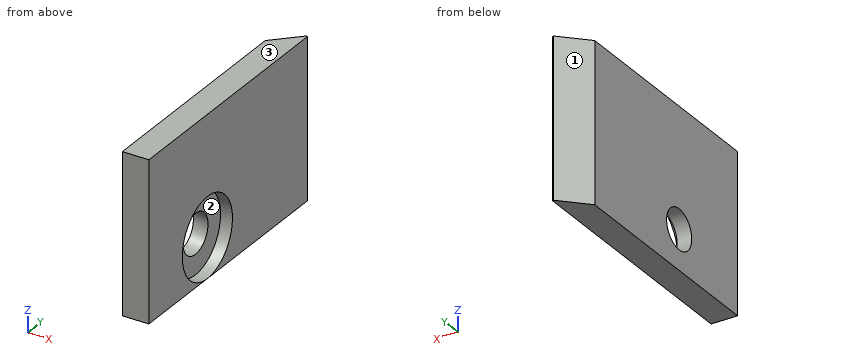
from build123d import *

# Parameters (mm, degrees)
CYLINDER3124_R               = 3
CYLINDER3124_DEPTH           = 3
COMPOUND1375_PLACEMENT_ANGLE = 90
CYLINDER3123_R               = 1.5
CYLINDER3123_DEPTH           = 12
CYLINDER3126_R               = 1.5
CYLINDER3126_DEPTH           = 4
BOX1133_W                    = 6
BOX1133_H                    = 6
BOX1133_DEPTH                = 2
COMPOUND1373_PLACEMENT_ANGLE = 90
BOX1134_W                    = 2
BOX1134_H                    = 19
BOX1134_DEPTH                = 12
CHAMFER182_SIZE              = 1.9


with BuildPart() as compound1375:
    # Cylinder3124 → Cylinder3124 (new body)
    with BuildSketch(Plane(origin=(1, 14, 6), x_dir=(1, 0, 0), z_dir=(0, 0, 1))):
        Circle(CYLINDER3124_R)
    extrude(amount=CYLINDER3124_DEPTH)


with BuildPart() as compound1375_1:
    # Compound1375 placement: moved
    add(compound1375.part.moved(Location((16.5, 73, 2))).rotate(Axis((16.5, 73, 2), (0, 1, 0)), COMPOUND1375_PLACEMENT_ANGLE))


with BuildPart() as obj1:
    # Cylinder3123 → Cylinder3123 (new body)
    with BuildSketch(Plane(origin=(1, 14, 6), x_dir=(1, 0, 0), z_dir=(0, 0, 1))):
        Circle(CYLINDER3123_R)
    extrude(amount=CYLINDER3123_DEPTH)


with BuildPart() as obj2:
    # Cylinder3126 → Cylinder3126 (new body)
    with BuildSketch(Plane(origin=(1, 14, -0.1), x_dir=(1, 0, 0), z_dir=(0, 0, 1))):
        Circle(CYLINDER3126_R)
    extrude(amount=CYLINDER3126_DEPTH)


with BuildPart() as compound1373:
    # Box1133 → Box1133 (new body)
    with BuildSketch(Plane(origin=(-2, 11, 4), x_dir=(1, 0, 0), z_dir=(0, 0, 1))):
        with Locations((3, 3)):
            Rectangle(BOX1133_W, BOX1133_H)
    extrude(amount=BOX1133_DEPTH)

    # Compound1373: union obj1, obj2
    add(obj1.part)
    add(obj2.part)


with BuildPart() as compound1373_1:
    # Compound1373 placement: moved
    add(compound1373.part.moved(Location((6, 73, 2))).rotate(Axis((6, 73, 2), (0, 1, 0)), COMPOUND1373_PLACEMENT_ANGLE))


with BuildPart() as chamfer182:
    # Box1134 → Box1134 (new body)
    with BuildSketch(Plane(origin=(21.4, 80, -2), x_dir=(1, 0, 0), z_dir=(0, 0, 1))):
        with Locations((1, 9.5)):
            Rectangle(BOX1134_W, BOX1134_H)
    extrude(amount=BOX1134_DEPTH)

    # Cut1268: cut Compound1373
    add(compound1373_1.part, mode=Mode.SUBTRACT)

    # Cut1269: cut Compound1375
    add(compound1375_1.part, mode=Mode.SUBTRACT)

    # Chamfer182
    chamfer182_edges = [chamfer182.edges().sort_by_distance(p)[0] for p in [
        (21.4, 99, 4),
    ]]
    chamfer(chamfer182_edges, length=CHAMFER182_SIZE)


with BuildPart() as chamfer182_1:
    # Chamfer182 placement: moved
    add(chamfer182.part.moved(Location((0.2, 3, 0))))


solid = chamfer182_1.part
The listing builds one solid part. Answer for the finished solid, in the listing's coordinates (mm). Face numbers are marked on the shaded views. Give positions to 0.01 mm unless a question says otherwise; leave off trailing zeros. Order: outer loops, then holes, each group sorted by start corner. A loop starts at its lowest first (then second) coordinate and runs counter-clockwise, first axis right, second up. Notation, with made-up numbers: (-31.5, 83) - (-9.5, 83) arc R22 cw to (-9.5, 102) - close; hole circle Ø4 at (-12, 16.5). An arc over 180 degrees is marked (long way). One line per item, written item: value. Start each with the question number.
1) Find the intervals of material crossed by L1, parallel to Z at x = 22.1, y = 90; L2, parallel to Y at x = 22.6, z = 1.5; L3, parallel to Y at x = 23.2, z = -1, in increasing order.
2) The mould has two halves that part along Y. Classify the marked faces 1, 2 and 3: released by +Y, released by -Y, zero draft, split by the parting line, or undercut.
3) Given pin 1 Ø5 at (y, z) = (90, 1) entering from +X; pin 2 Ø1 at (x, z) = (22, 1.5) entering from +Y, each flat-ended and moving along its own axis, determine where each tip first touches the part or whether it passes through.
4) A cutting plane is placed at A-A on x = 21.85. Give the vertices of the cut face in (y, z), then the cut area to 3 significant figures.
5) A cutting plane is placed at B-B on z = 5.5. Give the vertices of the cut face in (x, y).
Answer sheet:
1. L1: z = -2 to -0.5, 2.5 to 10
1. L2: y = 83 to 88.59, 91.41 to 101.1
1. L3: y = 83 to 87.76, 92.24 to 101.7
2. face 1: released by +Y
2. face 2: undercut
2. face 3: zero draft
3. pin 1: stops at x = 22.7
3. pin 2: stops at y = 101
4. outline: (83, -2) - (100.35, -2) - (100.35, 10) - (83, 10) - close; hole circle Ø3 at (90, 1)
4. area: 201 mm2
5. outline: (21.6, 83) - (23.6, 83) - (23.6, 102) - (23.5, 102) - (21.6, 100.1) - close
